Read the model definition and answer for the solid it produces. Units are mm, in the model's axes. A direction names the side the tool comes from. Round coordinates to 2 decimals unless told otherwise and drop trailing zeros. Loops run counter-clockwise (first coordinate to the right, second up) from the corner with the lowest first, then second, coordinate; pieces in that order, holes last. Notation, with made-up numbers: (67, 55.25) - (105, 55.25) arc R18 cw to (105, 60.25) - close; hole circle Ø2 at (-37.75, 41.25). An arc over 180 degrees is marked (long way). Use CSV: the item, a comma, the result in double quotes. Start each with the question number.
1. Consider line 1 along X through (y, z) = (0.25, 0.6); line 2 along Y through (x, z) = (0, 2.05); line 3 along X through (y, z) = (-2.5, 3.75). Determine where each line is inside the solid, lowest interval first.
2. Given pin 1 Ø2 at (y, z) = (1.5, 4.5) entering from +X; pin 2 Ø4.5 at (x, y) = (0, 0) entering from +Z; pin 3 Ø4 at (x, y) = (-193.5, -1) entering from -Z; pin 4 Ø3 at (x, z) = (-99.5, 3) entering from -Y, each flat-ended and moving along its own axis, determine where each tip first touches the part or whether it passes through.
3. A tool of negligible diameter and unlimited length cuts with its end or side. For faces 1 (the cylindrical face through (-76.52, -1.1, 2.96)), 2 (the flat face through (-81, -5, 3)), 3 (the flat face through (-79, 5, 3)), 4 (the cylindrical face through (5, 0, 3)), 5 (the flat face through (-186, 0, 2.9)), from which of +Z, -Z, +X, -X, +Y, -Y can it reach the whole face along a straight path? Write none if from no direction.
4. Find section B-B (z = 3.9). Give the vertices of the cut face in (x, y), and give its area (3 significant figures).
5. Determine the mould class of faces 6 (the flat face through (-185, 9, 3)), 7 (the flat face through (-124, 0, 6)), 8 (the flat face through (-185, -9, 3)), 9 (the cylindrical face through (-196.52, -1.1, 4.43)) for opening direction Y: +Y half, -Y half, draft (parallel to the pull), parting line (faces both ways), or undercut.
6. Find section C-C (x = -80). Give the vertices of the cut face in (y, z), and give its area (3 significant figures).
7. Find section D-D (x = -179). Give the vertices of the cut face in (y, z).
8. Find section A-A (y = 0). Give the vertices of the cut face in (x, z), and give its area (3 significant figures).
Autodesk Inventor part; units mm, degrees
ref_plane "YZ Plane" through (0, 0, 0) normal (1, 0, 0) x (0, 1, 0)
ref_plane "XZ Plane" through (0, 0, 0) normal (0, 1, 0) x (-1, 0, 0)
ref_plane "XY Plane" through (0, 0, 0) normal (0, 0, 1) x (1, 0, 0)
sketch "草圖1" plane through (0, 0, 0) normal (0, 0, 1) x (1, 0, 0)
  line L0 (-200, 0) -> (0, 0) construction
  line L1 (-200, -5) -> (0, -5)
  line L2 (0, 5) -> (-200, 5)
  arc A0 (-200, 5) -> (-200, -5) centre (-200, 0) ccw
  arc A1 (0, -5) -> (0, 5) centre (0, 0) ccw
  circle A2 centre (0, 0) radius 3.65
  circle A3 centre (-80, 0) radius 3.65
  circle A4 centre (-200, 0) radius 3.65
  point P0 (-100, 0)
  dimension "d0" = 200
  dimension "d1" = 10
  dimension "d3" = 7.3
  dimension "d27" = 7.3
  dimension "d47" = 7.3
extrude "擠出1" add sketch "草圖1" along normal blind 6 contours A0 L2 A1 L1 | A4
sketch "草圖4" plane through (0, 0, 0) normal (0, 0, -1) x (-1, 0, 0)
  line L0 (200, 0) -> (170.2, 0) construction
  line L1 (200, -9) -> (170.2, -9)
  line L2 (170.2, 9) -> (200, 9)
  arc A0 (200, -9) -> (200, 9) centre (200, 0) ccw
  arc A1 (170.2, 9) -> (170.2, -9) centre (170.2, 0) ccw
  arc A2 (200, -5) -> (200, 5) centre (200, 0) ccw
  circle A3 centre (170.2, 0) radius 0.6
  circle A4 centre (170.2, 0) radius 4.4
  circle A5 centre (200, 0) radius 6.65
  line L3 (169.8678, 4.3874) -> (199.4979, 6.631)
  line L4 (169.8678, -4.3874) -> (199.4979, -6.631)
  point P0 (0, 0)
  point P1 (185.1, 0)
  dimension "d31" = 9
  dimension "d36" = 1.2
  dimension "d37" = 29.8
  dimension "d42" = 8.8
  dimension "d44" = 13.3
extrude "擠出5" add sketch "草圖4" against normal blind 6 contours L1 A1 L2 A0 | A3 | A4 | A4 L3 A5 L4 | A5
extrude "擠出6" cut sketch "草圖4" against normal blind 2.9 contours A3 | A4 | A4 L3 A5 L4 | A5
extrude "擠出7" cut sketch "草圖1" along normal through all contours A4
fillet "圓角1" radius 5 2 edges at (-162.7167, 5, 3) (-162.7167, -5, 3)
properties part number "200_forservo"
Filled sheet:
1,line 1,"x = -209 to -206.65, -165.81 to -83.64, -76.36 to -3.64, 3.64 to 4.99"
1,line 2,"y = -5 to -3.65, 3.65 to 5"
1,line 3,"x = -208.65 to -202.66, -197.34 to -82.66, -77.34 to -2.66, 2.66 to 4.33"
2,pin 1,"stops at x = 4.97"
2,pin 2,"passes through"
2,pin 3,"stops at z = 2.9"
2,pin 4,"stops at y = -5"
3,face 1,"+Z, -Z"
3,face 2,"+Z, -Z, +X, -Y"
3,face 3,"+Z, -Z, +X, +Y"
3,face 4,"+Z, -Z, +X"
3,face 5,"-Z"
4,outline,"(-200, -9) - (-170.2, -9) arc R9 ccw to (-163.9, -6.43) arc R5 cw to (-160.4, -5) - (0, -5) arc R5 ccw to (0, 5) - (-160.4, 5) arc R5 cw to (-163.9, 6.43) arc R9 ccw to (-170.2, 9) - (-200, 9) arc R9 ccw to start; hole circle Ø7.3 at (-200, 0); hole circle Ø7.3 at (-80, 0); hole circle Ø7.3 at (0, 0)"
4,area,"2,320 mm²"
5,face 6,"+Y half"
5,face 7,"draft"
5,face 8,"-Y half"
5,face 9,"undercut"
6,outline,"(-5, 0) - (-3.65, 0) - (-3.65, 6) - (-5, 6) - close; (3.65, 0) - (5, 0) - (5, 6) - (3.65, 6) - close"
6,area,"16.2 mm²"
7,outline,"(-9, 0) - (-5.08, 0) - (-5.08, 2.9) - (5.08, 2.9) - (5.08, 0) - (9, 0) - (9, 6) - (-9, 6) - close"
8,outline,"(-209, 0) - (-206.65, 0) - (-206.65, 2.9) - (-203.65, 2.9) - (-203.65, 6) - (-209, 6) - close; (-196.35, 2.9) - (-165.8, 2.9) - (-165.8, 0) - (-83.65, 0) - (-83.65, 6) - (-196.35, 6) - close; (-76.35, 0) - (-3.65, 0) - (-3.65, 6) - (-76.35, 6) - close; (3.65, 0) - (5, 0) - (5, 6) - (3.65, 6) - close"
8,area,"1,060 mm²"
